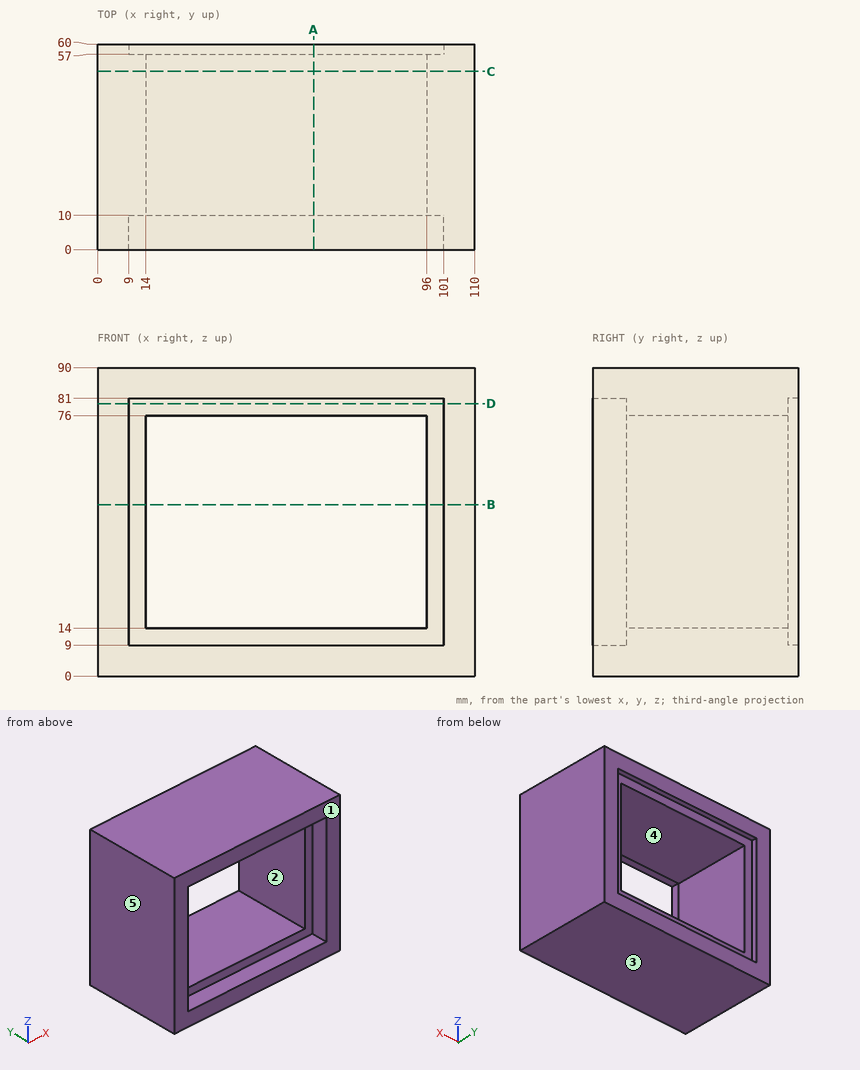
Here's the drawing with two shaded views (mm, measured from the low corner). I have some questions. A direction names the side the tool comes from. Give positions to 0.01 mm unless a question says otherwise; leave off trailing zeros. Write each loop counter-clockwise with the first axis right and the second up, starting at its lowest first coordinate (ties: lowest second). Pieces come first, ordered by that corner, then holes. Notation, with made-up numbers: (33, 1) -> (63, 1) arc R32 ccw to (63, 35) -> close; hole circle Ø6 at (2.25, 81.5). An arc over 180 degrees is marked (long way). Answer as a JSON object with one key per item and string values. Group by question number.
Item 1: Suppose I cut it at D-D (z = 79.5). Please give me the cut outline in (x, y).
Item 2: Suppose I cut it at C-C (y = 52). Please give me the cut outline in (x, z).
Item 3: For the marked faces 4 and 5, which set-ups out of +Z, -Z, +X, -X, +Y, -Y let a thin tool reach every point of the face, with its end or its side?
Item 4: Please list where these lines run through material, in increasing order: line 1 (Z direction, x = 47.5, y = 19.5); line 2 (X direction, y = 23, z = 68); line 3 (X direction, y = 9.5, z = 27). Write a range as [from, to].
Item 5: Suppose I cut it at A-A (x = 63). Please give me the cut outline in (y, z).
Item 6: I'm going to push a flat-ended pin straight in: P1, Ø2, axis at x = 77, z = 10.5, coming from the -Y side. Where does the tip first touch, or does it pass through?
Item 7: We'd pull the mould along Z, two halves only. Please class the marked faces 1, 2 and 3: +Z half, -Z half, draft (parallel to the pull), parting line (faces both ways), or undercut.
Item 8: Suppose I cut it at B-B (z = 50). Please give me the cut outline in (x, y).
Findings:
{
 "1": {"outline": "(0, 0) -> (9, 0) -> (9, 10) -> (101, 10) -> (101, 0) -> (110, 0) -> (110, 60) -> (101, 60) -> (101, 57) -> (9, 57) -> (9, 60) -> (0, 60) -> close"},
 "2": {"outline": "(0, 0) -> (110, 0) -> (110, 90) -> (0, 90) -> close; hole (14, 14) -> (96, 14) -> (96, 76) -> (14, 76) -> close"},
 "3": {"face 4": "+Y, -Y", "face 5": "+Z, -Z, -X, +Y, -Y"},
 "4": {"line 1": "z = [0, 14], [76, 90]", "line 2": "x = [0, 14], [96, 110]", "line 3": "x = [0, 9], [101, 110]"},
 "5": {"outline": "(0, 0) -> (60, 0) -> (60, 9) -> (57, 9) -> (57, 14) -> (10, 14) -> (10, 9) -> (0, 9) -> close; (0, 81) -> (10, 81) -> (10, 76) -> (57, 76) -> (57, 81) -> (60, 81) -> (60, 90) -> (0, 90) -> close"},
 "6": {"P1": "stops at y = 10"},
 "7": {"face 1": "draft", "face 2": "undercut", "face 3": "-Z half"},
 "8": {"outline": "(0, 0) -> (9, 0) -> (9, 10) -> (14, 10) -> (14, 57) -> (9, 57) -> (9, 60) -> (0, 60) -> close; (96, 10) -> (101, 10) -> (101, 0) -> (110, 0) -> (110, 60) -> (101, 60) -> (101, 57) -> (96, 57) -> close"}
}
